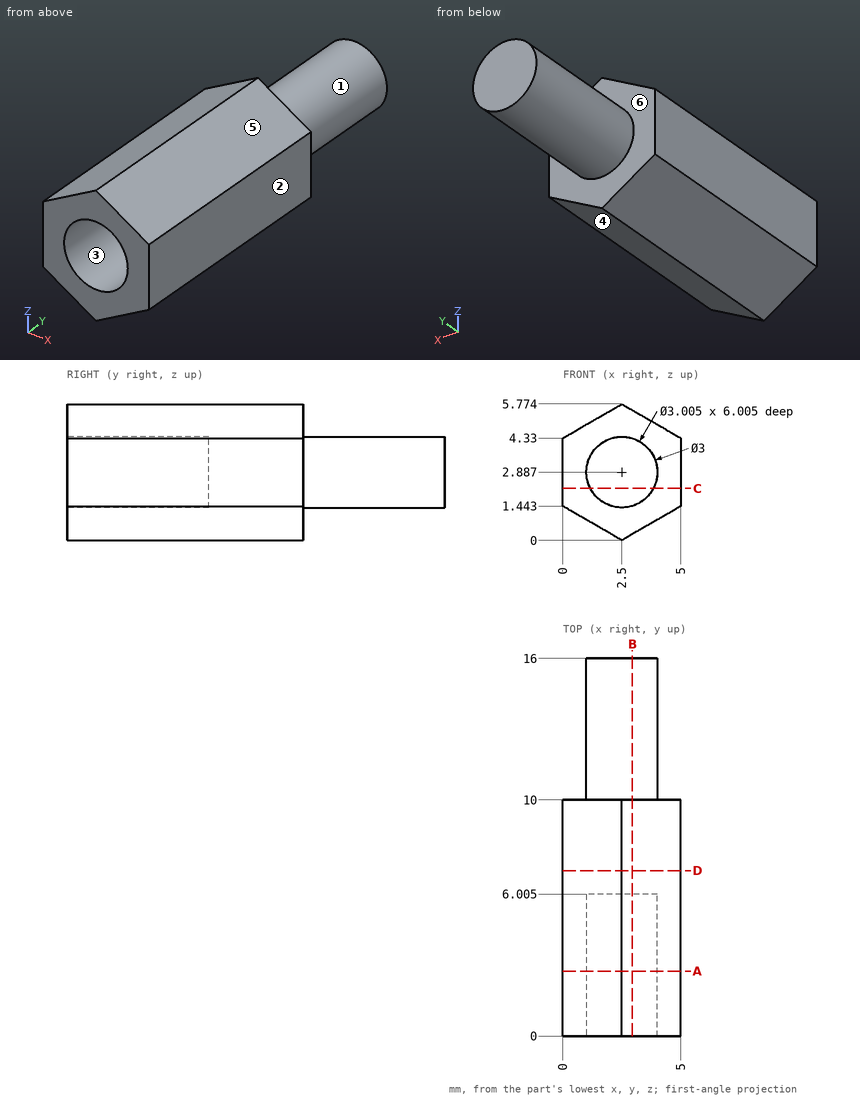
Geometry check sheet. Reference: drawing and pictorial views, mm from the part's lowest x, y, z. A direction names the side the tool comes from. Give positions to 0.01 mm unless a question says otherwise; leave off trailing zeros. Loops run counter-clockwise (first coordinate to the right, second up) from the corner with the lowest first, then second, coordinate; pieces in that order, holes last. Notation, with made-up numbers: M 24.5,-38.75 L 73.5,-38.75 A22 cw 73.5,-28.75 Z; hole C 1.5,22.5 d7. An arc over 180 degrees is marked long. Use a Markdown table: item, result. Add a question column.
Q1. Sectioned sample at B-B, the plane x = 2.95. Record the cut outline in (y, z) (1 decimal).
Q2. Scan lines: line 1 along Y through (x, z) = (2.65, 1.45) (1 decimal); line 2 along Z through (x, y) = (1.45, 1.5) (1 decimal); line 3 along Y through (x, z) = (0.85, 1.8). Record each from-to range of solid material in increasing order. Write a range as [from, to].
Q3. Sectioned sample at D-D, the plane y = 7. Record the cut outline in (x, z).
Q4. Sectioned sample at C-C, the plane z = 2.2. Record the cut outline in (x, y) (1 decimal).
Q5. Tool access check on the marked faces 5 and 6. Record the directions out of +Z, -Z, +X, -X, +Y, -Y that give a thin tool (end or side, any length) a straight path to the whole face; none if there is none.
Q6. Mould release check, pull along Z, two halves, no side actions. Record for the marked faces 1, 2, 3 and 4: pulls with the +Z half, pulls with the -Z half, needs draft (parallel to the pull), parting line crosses it, or undercut.
Q7. Sectioned sample at A-A, the plane y = 2.75. Record the cut outline in (x, z) (1 decimal).
Q8. Go/stop test with a flat-tipped pin: pin 1 (2 mm diameter, centred on x = 1.5, z = 1.5, fed in from -Y). Record where the tip stops, or that it passes through.
Verdict:
| question | item | result |
|---|---|---|
| 1 | outline | M 0,0.3 L 10,0.3 L 10,1.5 L 16,1.5 L 16,4.3 L 10,4.3 L 10,5.5 L 0,5.5 L 0,4.3 L 6,4.3 L 6,1.5 L 0,1.5 Z |
| 2 | line 1 | [6, 16] |
| 2 | line 2 | [0.6, 1.8], [4, 5.2] |
| 2 | line 3 | [0, 10] |
| 3 | outline | M 0,1.44 L 2.5,0 L 5,1.44 L 5,4.33 L 2.5,5.77 L 0,4.33 Z |
| 4 | outline | M 0,0 L 1.2,0 L 1.2,6 L 3.8,6 L 3.8,0 L 5,0 L 5,10 L 3.8,10 L 3.8,16 L 1.2,16 L 1.2,10 L 0,10 Z |
| 5 | face 5 | +Z, +X, +Y, -Y |
| 5 | face 6 | +Y |
| 6 | face 1 | parting line crosses it |
| 6 | face 2 | needs draft |
| 6 | face 3 | undercut |
| 6 | face 4 | pulls with the -Z half |
| 7 | outline | M 0,1.4 L 2.5,0 L 5,1.4 L 5,4.3 L 2.5,5.8 L 0,4.3 Z; hole C 2.5,2.9 d3 |
| 8 | pin 1 | y = 0 |
